The model under review builds one solid part; all positions refer to its coordinate system, in mm. Face numbers are marked on the shaded views. A direction names the side the tool comes from. Give positions to 0.01 mm unless a question says otherwise; leave off trailing zeros. Loops run counter-clockwise (first coordinate to the right, second up) from the corner with the lowest first, then second, coordinate; pieces in that order, holes last. Notation, with made-up numbers: M -2.5,62 L 32.5,62 A28 ccw 32.5,84 Z; hole C -24,-36 d10. An arc over 180 degrees is marked long. Return JSON: item names as keys, results as strings.
Autodesk Inventor part; units mm, degrees
ref_plane "YZ Plane" through (0, 0, 0) normal (1, 0, 0) x (0, 1, 0)
ref_plane "XZ Plane" through (0, 0, 0) normal (0, 1, 0) x (-1, 0, 0)
ref_plane "XY Plane" through (0, 0, 0) normal (0, 0, 1) x (1, 0, 0)
sketch "Boceto1" plane through (0, 0, 0) normal (0, 1, 0) x (-1, 0, 0)
  circle A0 centre (0, 0) radius 1
  dimension "d0" = 2
extrude "Extrusión1" add sketch "Boceto1" along normal blind 7
sketch "Boceto2" plane through (0, 7, 0) normal (0, 1, 0) x (1, 0, 0)
  circle A0 centre (0, 0) radius 1.5
  dimension "d3" = 3
extrude "Extrusión2" add sketch "Boceto2" along normal blind 2
fillet "Empalme1" radius 0.1 3 edges at (1, 0, 0) (-1.5, 7, 0) (-1.5, 9, 0)
properties part number "Tornillo 1"
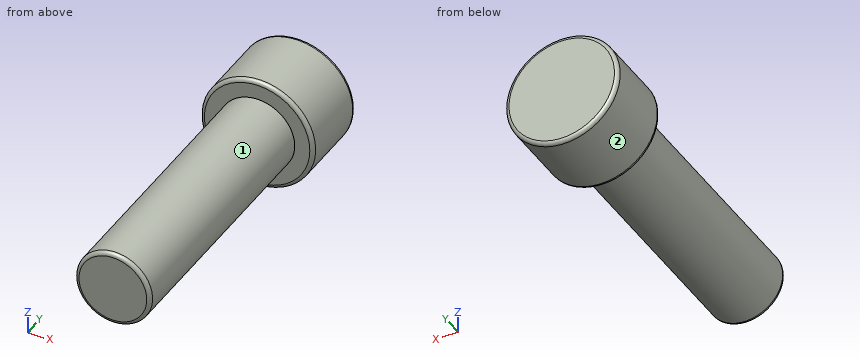
1) Consider section C-C on y = 8.75. Write out the cut boundary in (x, z), then the cut area to 3 significant figures.
From the geometry:
{"outline": "C 0,0 d3", "area": "7.07 mm²"}
2) Wall thickness on L1, parallel to Y at x = -0.85, z = -0.95; L2, parallel to X at y = 8, z = -0.25; L3, parallel to Y at x = 0.3, z = -0.9: over which ranges is each line inside the solid? List them lowest first. Write a range as from..to.
From the geometry:
{"L1": "7..9", "L2": "-1.48..1.48", "L3": "0.01..9"}
3) Consider section B-B on x = 0. Write out the cut boundary in (y, z), then the cut area to 3 significant figures.
From the geometry:
{"outline": "M 0,-0.9 A0.1 ccw 0.1,-1 L 7,-1 L 7,-1.4 A0.1 ccw 7.1,-1.5 L 8.9,-1.5 A0.1 ccw 9,-1.4 L 9,1.4 A0.1 ccw 8.9,1.5 L 7.1,1.5 A0.1 ccw 7,1.4 L 7,1 L 0.1,1 A0.1 ccw 0,0.9 Z", "area": "20.0 mm²"}
4) Consider section A-A on z = 0. Write out the cut boundary in (x, y), then the cut area to 3 significant figures.
From the geometry:
{"outline": "M -1.5,7.1 A0.1 ccw -1.4,7 L -1,7 L -1,0.1 A0.1 ccw -0.9,0 L 0.9,0 A0.1 ccw 1,0.1 L 1,7 L 1.4,7 A0.1 ccw 1.5,7.1 L 1.5,8.9 A0.1 ccw 1.4,9 L -1.4,9 A0.1 ccw -1.5,8.9 Z", "area": "20.0 mm²"}
5) Consider section D-D on y = 5.25. Write out the cut boundary in (x, z).
From the geometry:
{"outline": "C 0,0 d2"}
6) Tool access review of the marked faces 1 and 2: name each direction out of +Z, -Z, +X, -X, +Y, -Y from which nothing blocks a thin tool from reaching the whole face with its end or side.
From the geometry:
{"face 1": "-Y", "face 2": "+Y, -Y"}
